Input: part model. Units: mm. Frame: model coordinates. A direction names the side the tool comes from. Round coordinates to 2 decimals unless told otherwise and drop trailing zeros. Loops run counter-clockwise (first coordinate to the right, second up) from the corner with the lowest first, then second, coordinate; pieces in that order, holes last. Notation, with made-up numbers: M 89.25,55 L 103.25,55 A19 ccw 103.25,87 Z; hole C 42.25,87.5 d11. An arc over 180 degrees is marked long. Return JSON: item names as keys, results as strings. Group by question number.
1) Section C-C (z = -4). Output: boundary loops of the cut face in (x, y), plus the area to 3 significant figures.
2) Section A-A (z = -13.25). Count the separate pieces of the cut face and the enclosed holes in it, plus the area to 3 significant figures.
3) Section B-B (x = 35). Output: boundary loops of the cut face in (y, z).
4) Contact query for a flat-ended pin moving along its axis: P1, Ø3, axis at x = 52, y = 6.5, coming from the -Z side. Output: stop coordinate, or through.
5) Section D-D (y = 8). Output: boundary loops of the cut face in (x, z).
6) Mould query, pull axis X, two halves, no side actions, for faces 1 (the face through (-4, 12, -9)), 2 (the face through (71, 16, -11)), 3 (the face through (32.3, -0.2, -22)). Classes: +X half, -X half, draft (parallel to the pull), parting line (faces both ways), or undercut.
7) Access query for faces 4 (the face through (5.766, -1.521, -9.115)), 5 (the face through (-1, 17, -11)), 6 (the face through (-3, -1, -10)). Directions: +Z, -Z, +X, -X, +Y, -Y. A direction counts if a zero-diameter tool reaches every point of the face in a straight line with its end or side. Return the directions, or none.
8) Material intervals for line 1 (Y direction, x = 65.5, z = -13.5); line 2 (X direction, y = 2.5, z = -4); line 3 (X direction, y = 13, z = -6.25), sorted ascending. Write a range as from..to.
from build123d import *

# Parameters (mm, degrees)
SKETCH_1_W               = 70
SKETCH_1_H               = 20
EXTRUDE_1_DEPTH          = 3
SKETCH_2_W               = 78
SKETCH_2_H               = 30
EXTRUDE_2_DEPTH          = 3
SKETCH_4_W               = 16
SKETCH_4_H               = 12
SKETCH_4_W_2             = 9.1
SKETCH_4_H_2             = 6.5
EXTRUDE_3_DEPTH          = 22
SKETCH_5_W               = 46
SKETCH_5_H               = 3
EXTRUDE_4_DEPTH          = 22
EXTRUDE_5_DEPTH          = 22
CHAMFER_1_SIZE           = 3
CUT_EXTRUDE_1_DEPTH      = 82.786306922
CUT_EXTRUDE_1_DEPTH_BACK = 82.786306922
SKETCH_10_R              = 2.5
SKETCH_11_R              = 1.65
CUT_EXTRUDE_2_DEPTH      = 10


with BuildPart() as part:
    # 草图1 → 凸台-拉伸1 (new body)
    with BuildSketch(Plane.XY):
        with Locations((35, 10)):
            Rectangle(SKETCH_1_W, SKETCH_1_H)
    extrude(amount=EXTRUDE_1_DEPTH)

    # 草图2 → 凸台-拉伸2 (add)
    with BuildSketch(Plane.XY.offset(3)):
        with Locations((35, 12)):
            Rectangle(SKETCH_2_W, SKETCH_2_H)
    extrude(amount=-EXTRUDE_2_DEPTH)

    # 草图4 → 凸台-拉伸3 (add)
    with BuildSketch(Plane(origin=(0, 0, 0), x_dir=(-1, 0, 0), z_dir=(0, 0, -1))):
        with Locations((-66, 3)):
            Rectangle(SKETCH_4_W, SKETCH_4_H)
        with Locations((-65.45, 3.25)):
            Rectangle(SKETCH_4_W_2, SKETCH_4_H_2, mode=Mode.SUBTRACT)
    extrude_3 = extrude(amount=EXTRUDE_3_DEPTH)

    # 镜向1: 凸台-拉伸3 across plane
    add(extrude_3.mirror(Plane(origin=(35, 0, 0), x_dir=(0, 0, 1), z_dir=(1, 0, 0))))

    # 草图5 → 凸台-拉伸4 (add)
    with BuildSketch(Plane(origin=(0, 0, 0), x_dir=(-1, 0, 0), z_dir=(0, 0, -1))):
        with Locations((-35, -1.5)):
            Rectangle(SKETCH_5_W, SKETCH_5_H)
    extrude(amount=EXTRUDE_4_DEPTH)

    # 草图6 → 凸台-拉伸5 (add)
    with BuildSketch(Plane(origin=(0, 0, 0), x_dir=(-1, 0, 0), z_dir=(0, 0, -1))):
        Polygon((4, 27), (-74, 27), (-74, 24), (-74, 9), (-71, 9), (-71, 24), (1, 24), (1, 9), (4, 9), (4, 24), align=None)
    extrude(amount=EXTRUDE_5_DEPTH)

    # 倒角1
    chamfer_1_edges = [part.edges().sort_by_distance(p)[0] for p in [
        (-4, -3, -9.5),
        (-4, 27, -9.5),
        (74, 27, -9.5),
        (74, -3, -9.5),
    ]]
    chamfer(chamfer_1_edges, length=CHAMFER_1_SIZE)

    # 草图10 → 切除-拉伸1 (cut, two sides: drawn at the far end of the back side and taken through both)
    with BuildSketch(Plane.XZ.offset(-24).offset(-CUT_EXTRUDE_1_DEPTH_BACK)):
        with Locations((35, -13.25)):
            Circle(SKETCH_10_R)
    extrude(amount=CUT_EXTRUDE_1_DEPTH + CUT_EXTRUDE_1_DEPTH_BACK, mode=Mode.SUBTRACT)

    # 草图11 → 切除-拉伸2 (cut, symmetric)
    with BuildSketch(Plane.XZ.offset(-6.5)):
        with Locations(Location((4.55, -8, 0), (0, 0, 180))):
            Circle(SKETCH_11_R)
    cut_extrude_2 = extrude(amount=CUT_EXTRUDE_2_DEPTH, both=True, mode=Mode.SUBTRACT)

    # 镜向2: 切除-拉伸2 across plane
    add(cut_extrude_2.mirror(Plane(origin=(35, 0, 0), x_dir=(0, 0, 1), z_dir=(1, 0, 0))), mode=Mode.SUBTRACT)


solid = part.part
Returned:
{
 "1": {"outline": "M -4,0 L -1,-3 L 71,-3 L 74,0 L 74,24 L 71,27 L -1,27 L -4,24 Z; hole M -1,9 L 12,9 L 12,0 L 58,0 L 58,9 L 71,9 L 71,24 L -1,24 Z; hole M 0,0 L 9.1,0 L 9.1,6.5 L 0,6.5 Z; hole M 60.9,0 L 70,0 L 70,6.5 L 60.9,6.5 Z", "area": "710 mm^2"},
 "2": {"separate pieces": "2", "enclosed holes": "2", "area": "680 mm^2"},
 "3": {"outline": "M -3,-22 L 0,-22 L 0,-15.75 L -3,-15.75 Z; M -3,-10.75 L 0,-10.75 L 0,0 L 24,0 L 24,-10.75 L 27,-10.75 L 27,3 L -3,3 Z; M 24,-22 L 27,-22 L 27,-15.75 L 24,-15.75 Z"},
 "4": {"P1": "stops at z = 0"},
 "5": {"outline": "M -4,-22 L 12,-22 L 12,0 L 58,0 L 58,-22 L 74,-22 L 74,3 L -4,3 Z; hole C 4.55,-8 d3.3; hole C 65.45,-8 d3.3"},
 "6": {"face 1": "-X half", "face 2": "undercut", "face 3": "draft"},
 "7": {"face 4": "-Y", "face 5": "-Z", "face 6": "+Z, -Z, -X, -Y"},
 "8": {"line 1": "y = -3..0, 6.5..9, 24..27", "line 2": "x = -4..0, 9.1..12, 58..60.9, 70..74", "line 3": "x = -4..-1, 71..74"}
}
